For this review, take the finished solid that the model builds, in its own axes (mm). A direction names the side the tool comes from. Give positions to 0.01 mm unless a question says otherwise; leave off trailing zeros. Write each loop counter-clockwise with the first axis right and the second up, starting at its lowest first coordinate (ties: lowest second). Pieces come first, ordered by that corner, then holes. Notation, with made-up numbers: M -21.75,48 L 30.25,48 A20 cw 30.25,54 Z; hole C 83,42.25 d4. An arc over 180 degrees is marked long. Write item = value, one per line.
```python
from build123d import *

# Parameters (mm, degrees)
SKETCH1_R           = 1.6
BOSS_EXTRUDE1_DEPTH = 4.6
CUT_EXTRUDE4_DEPTH  = 1.4


with BuildPart() as part:
    # Sketch1 → Boss-Extrude1 (new body)
    with BuildSketch(Plane.XY):
        with BuildLine():
            Line((-33.815617771, -15.817972293), (-13.905712582, 19.727465886))
            ThreePointArc((-13.905712582, 19.727465886), (-12.438375238, 21.223732505), (-10.415875199, 21.77271909))
            Line((-10.415875199, 21.77271909), (30.325780388, 21.77271909))
            ThreePointArc((30.325780388, 21.77271909), (33.776793804, 19.795219128), (33.815617771, 15.817972293))
            Line((33.815617771, 15.817972293), (13.905712582, -19.727465886))
            ThreePointArc((13.905712582, -19.727465886), (12.438375238, -21.223732505), (10.415875199, -21.77271909))
            Line((10.415875199, -21.77271909), (-30.325780388, -21.77271909))
            ThreePointArc((-30.325780388, -21.77271909), (-33.776793804, -19.795219128), (-33.815617771, -15.817972293))
        make_face()
        with Locations((-4.949747468, 4.949747468)):
            Circle(SKETCH1_R, mode=Mode.SUBTRACT)
        with Locations((4.949747468, 4.949747468)):
            Circle(SKETCH1_R, mode=Mode.SUBTRACT)
        with Locations((4.949747468, -4.949747468)):
            Circle(SKETCH1_R, mode=Mode.SUBTRACT)
        with Locations((-4.949747468, -4.949747468)):
            Circle(SKETCH1_R, mode=Mode.SUBTRACT)
    extrude(amount=BOSS_EXTRUDE1_DEPTH)

    # Sketch5 → Cut-Extrude4 (cut)
    with BuildSketch(Plane.XY.offset(4.6)):
        with BuildLine():
            Line((11.637318283, -18.456880469), (31.547223472, 17.088557711))
            ThreePointArc((31.547223472, 17.088557711), (31.533635084, 18.480594103), (30.325780388, 19.17271909))
            Line((30.325780388, 19.17271909), (-10.415875199, 19.17271909))
            ThreePointArc((-10.415875199, 19.17271909), (-11.123750213, 18.980573785), (-11.637318283, 18.456880469))
            Line((-11.637318283, 18.456880469), (-31.547223472, -17.088557711))
            ThreePointArc((-31.547223472, -17.088557711), (-31.533635084, -18.480594103), (-30.325780388, -19.17271909))
            Line((-30.325780388, -19.17271909), (10.415875199, -19.17271909))
            ThreePointArc((10.415875199, -19.17271909), (11.123750213, -18.980573785), (11.637318283, -18.456880469))
        make_face()
    extrude(amount=-CUT_EXTRUDE4_DEPTH, mode=Mode.SUBTRACT)


solid = part.part
```
1. For line 1 along Y through (x, z) = (-6.5, 3.9); line 2 along X through (y, z) = (6, 1.85); line 3 along Z through (x, y) = (7.5, 0.5), list the stretches that pass through material, from the lowest coordinate up. Write a range as from..to.
Responses:
line_1 = -21.77..-19.17, 19.17..21.77
line_2 = -21.59..-6.16, -3.74..3.74, 6.16..28.32
line_3 = 0..3.2
2. We need section C-C, the plane y = 2. Write out the cut boundary in (x, z), then the cut area to 3 significant figures.
Responses:
outline = M -23.84,0 L 26.08,0 L 26.08,4.6 L 23.1,4.6 L 23.1,3.2 L -20.86,3.2 L -20.86,4.6 L -23.84,4.6 Z
area = 168 mm2
3. Insertion check: P1, Ø4, axis at x = 4.95, y = -4.95, coming from the +Z side; P2, Ø1.5, axis at y = -10.5, z = 2.5, coming from the +X side. Each pin has a flat end and moves straight along its axis. Give the tip position at first contact, or say it passes through.
Responses:
P1 = 3.2
P2 = 19.49
4. We need section A-A, the plane z = 1.15. Write out the cut boundary in (x, y), then the cut area to 3 significant figures.
Responses:
outline = M -33.82,-15.82 A4 ccw -30.33,-21.77 L 10.42,-21.77 A4 ccw 13.91,-19.73 L 33.82,15.82 A4 ccw 30.33,21.77 L -10.42,21.77 A4 ccw -13.91,19.73 Z; hole C -4.95,-4.95 d3.2; hole C -4.95,4.95 d3.2; hole C 4.95,-4.95 d3.2; hole C 4.95,4.95 d3.2
area = 2,120 mm2
5. Machinability: for faces 1 (the face through (-21.453, 0.933, 3.91)), 2 (the face through (-5.3, 3.39, 1.58)), which of the approach directions +Z, -Z, +X, -X, +Y, -Y give a long, thin tool a straight path to every point of the face, cutting with its end or side? Answer none if there is none.
Responses:
face_1 = +Z
face_2 = +Z, -Z
6. We need section B-B, the plane x = -26.5. Write out the cut boundary in (y, z).
Responses:
outline = M -21.77,0 L -2.76,0 L -2.76,4.6 L -8.08,4.6 L -8.08,3.2 L -19.17,3.2 L -19.17,4.6 L -21.77,4.6 Z
7. The part is to be moulded in two halves that separate along X. For faces 3 (the face through (-10, -21.773, 2)), 4 (the face through (33.747, 19.845, 2.268)), 5 (the face through (-24, 1.71, 2.27)), 6 (the face through (-31.544, -18.463, 3.91)), say which applies: +X half, -X half, draft (parallel to the pull), parting line (faces both ways), or undercut.
Responses:
face_3 = draft
face_4 = +X half
face_5 = -X half
face_6 = undercut
